For this review, take the finished solid that the model builds, in its own axes (mm). A direction names the side the tool comes from. Give positions to 0.01 mm unless a question says otherwise; leave off trailing zeros. Order: outer loops, then holes, each group sorted by start corner. A loop starts at its lowest first (then second) coordinate and runs counter-clockwise, first axis right, second up. Notation, with made-up numbers: M -30,89 L 11,89 A5 cw 11,94 Z; hole C 43,76 d11. An arc over 180 degrees is marked long. Use CSV: the item, a comma, the result in double quotes. Start each with the question number.
(1) Consider section A-A (y = 0). Write out the cut boundary in (x, z) (3 decimals).
(2) Wall thickness on L1, parallel to Z at x = -0.25, y = -6.75 (3 decimals); L2, parallel to Y at x = -3, z = -6.25; L3, parallel to Y at x = 4, z = -11.75: over which ranges is each line inside the solid? List them lowest first. Write a range as from..to.
(3) Consider section C-C (z = -6.35). Write out the cut boundary in (x, y) (3 decimals), and give its area (3 significant figures).
(4) Consider section D-D (z = -4). Write out the cut boundary in (x, y).
(5) Clearance check with a flat-ended pin moving along its axis: P1, Ø4, axis at y = 8, z = -5.5, coming from the +X side. State where the tip first meets the part, or that it passes through.
(6) Tool access review of faces 1 (the face through (-0.13, 15.24, -6.21)), 2 (the face through (0, 0, -1.905)): name each direction out of +Z, -Z, +X, -X, +Y, -Y from which nothing blocks a thin tool from reaching the whole face with its end or side.
(7) Consider section B-B (x = 0.75). Write out the cut boundary in (y, z) (3 decimals).
(8) Draft analysis for pull direction Z (two halves, no side actions). For faces 3 (the face through (-9.271, 5, -11)), 4 (the face through (0, 0, -10.795)), 5 (the face through (0, 0, 0)), state which applies: pulls with the +Z half, pulls with the -Z half, needs draft (parallel to the pull), parting line crosses it, or undercut.
```python
from build123d import *

# Parameters (mm, degrees)
SKETCH1_W           = 18.542
SKETCH1_H           = 17.78
BOSS_EXTRUDE4_DEPTH = 1.905
SKETCH4_W           = 18.542
SKETCH4_H           = 17.78
BOSS_EXTRUDE5_DEPTH = 1.905
BOSS_EXTRUDE6_DEPTH = 18.542


with BuildPart() as part:
    # Sketch1 → Boss-Extrude4 (new body)
    with BuildSketch(Plane.XY):
        Rectangle(SKETCH1_W, SKETCH1_H)
    extrude(amount=-BOSS_EXTRUDE4_DEPTH)



with BuildPart() as body_2:
    # Sketch4 → Boss-Extrude5 (new body)
    with BuildSketch(Plane.XY.offset(-12.7)):
        Rectangle(SKETCH4_W, SKETCH4_H)
    extrude(amount=BOSS_EXTRUDE5_DEPTH)


with BuildPart() as part_1:
    add(part.part)

    add(body_2.part)  # Boss-Extrude6 merges body 2
    # Sketch6 → Boss-Extrude6 (add)
    with BuildSketch(Plane.ZY.offset(9.271)):
        with BuildLine():
            Line((-12.7, 8.89), (-10.795, 8.89))
            ThreePointArc((-10.795, 8.89), (-6.35, 13.335), (-1.905, 8.89))
            Line((-1.905, 8.89), (0, 8.89))
            ThreePointArc((0, 8.89), (-6.35, 15.24), (-12.7, 8.89))
        make_face()
    extrude(amount=-BOSS_EXTRUDE6_DEPTH)


solid = part_1.part
```
Check result:
1,outline,"M -9.271,-12.7 L 9.271,-12.7 L 9.271,-10.795 L -9.271,-10.795 Z; M -9.271,-1.905 L 9.271,-1.905 L 9.271,0 L -9.271,0 Z"
2,L1,"z = -12.7..-10.795, -1.905..0"
2,L2,"y = 13.33..15.24"
2,L3,"y = -8.89..12.23"
3,outline,"M -9.271,13.335 L 9.271,13.335 L 9.271,15.24 L -9.271,15.24 Z"
3,area,"35.3 mm^2"
4,outline,"M -9.27,12.66 L 9.27,12.66 L 9.27,14.79 L -9.27,14.79 Z"
5,P1,"passes through"
6,face 1,"+X, -X, +Y"
6,face 2,"+X, -X, -Y"
7,outline,"M -8.89,-12.7 L 8.89,-12.7 A6.35 ccw 8.89,0 L -8.89,0 L -8.89,-1.905 L 8.89,-1.905 A4.445 cw 8.89,-10.795 L -8.89,-10.795 Z"
8,face 3,"needs draft"
8,face 4,"undercut"
8,face 5,"pulls with the +Z half"
